from build123d import *

# Parameters (mm, degrees)
SKETCH_1_W      = 33
SKETCH_1_H      = 16
SKETCH_1_R      = 1.7
EXTRUDE_1_DEPTH = 5
EXTRUDE_2_DEPTH = 2.65
SKETCH_3_W      = 0.8
SKETCH_3_H      = 5
EXTRUDE_3_DEPTH = 10
CHAMFER_1_SIZE  = 0.6


with BuildPart() as part:
    # 草图1 → 凸台-拉伸1 (new, symmetric)
    with BuildSketch(Plane(origin=(0, 0, 0), x_dir=(1, 0, 0), z_dir=(0, 1, 0))):
        Rectangle(SKETCH_1_W, SKETCH_1_H)
        with Locations(Location((-11.1, 5, 0), (0, 0, 270))):
            Circle(SKETCH_1_R, mode=Mode.SUBTRACT)
        with Locations(Location((11.1, -5, 0), (0, 0, 270))):
            Circle(SKETCH_1_R, mode=Mode.SUBTRACT)
    extrude(amount=EXTRUDE_1_DEPTH, both=True)

    # 草图2 → 凸台-拉伸2 (add, symmetric)
    with BuildSketch(Plane(origin=(0, 0, 0), x_dir=(1, 0, 0), z_dir=(0, 1, 0))):
        with BuildLine():
            Line((3.236985687, -9.8), (-13.498945121, -9.8))
            Line((-13.498945121, -9.8), (-13.498945121, -10.3))
            Line((-13.498945121, -10.3), (-2.457771256, -10.3))
            Line((-2.457771256, -10.3), (-13.404349416, -11.402516894))
            Line((-13.404349416, -11.402516894), (-13.354243938, -11.9))
            Line((-13.354243938, -11.9), (6.231752422, -9.92733863))
            Line((6.231752422, -9.92733863), (6.231752422, -4.606941304))
            ThreePointArc((6.231752422, -4.606941304), (4.679221154, -3.232884233), (3.236985687, -4.72229453))
            Line((3.236985687, -4.72229453), (3.236985687, -9.8))
        make_face()
    extrude(amount=EXTRUDE_2_DEPTH, both=True)

    # 草图3 → 凸台-拉伸3 (add)
    with BuildSketch(Plane(origin=(16.5, 0, 0), x_dir=(0, 0, -1), z_dir=(1, 0, 0))):
        with Locations((-3.8, 0)):
            Rectangle(SKETCH_3_W, SKETCH_3_H)
        Rectangle(SKETCH_3_W, SKETCH_3_H)
        with Locations((3.8, 0)):
            Rectangle(SKETCH_3_W, SKETCH_3_H)
    extrude(amount=EXTRUDE_3_DEPTH)

    # 倒角1
    chamfer_1_edges = [part.edges().sort_by_distance(p)[0] for p in [
        (26.5, -2.5, 3.8),
        (26.5, 2.5, 3.8),
        (26.5, -2.5, 0),
        (26.5, 2.5, 0),
        (-16.5, 0, -8),
        (26.5, -2.5, -3.8),
        (16.5, 0, -8),
        (26.5, 2.5, -3.8),
        (16.5, 0, 8),
        (-16.5, 0, 8),
    ]]
    chamfer(chamfer_1_edges, length=CHAMFER_1_SIZE)


solid = part.part
Source: CAD feature listing. Evaluate the final solid. Frame: model axes, mm. A direction names the side the tool comes from. Round coordinates to 2 decimals unless told otherwise and drop trailing zeros. Order: outer loops, then holes, each group sorted by start corner. A loop starts at its lowest first (then second) coordinate and runs counter-clockwise, first axis right, second up. Notation, with made-up numbers: (-19.5, 42.5) - (5.5, 42.5) arc R20 ccw to (5.5, 65.5) - close; hole circle Ø7 at (32.25, 40.5). An arc over 180 degrees is marked (long way). Use a Markdown table: item, result. Add a question column.
1. Section query D-D (z = 5). Return the cut outline in (x, y).
2. Section query A-A (x = 24.5). Return the cut outline in (y, z).
3. Section query B-B (x = 11.1). Return the cut outline in (y, z), then the cut area to 3 significant figures.
4. Section query C-C (y = 0.5). Give the number of separate pieces and of enclosed holes in the cut face, then the cut area to 3 significant figures.
5. First-contact query: pin 1 (0.6 mm diameter, centred on y = 1.5, z = 10, fed in from -X); pin 2 (1.5 mm diameter, centred on x = 21, y = 0.5, fed in from +Z); pin 3 (0.9 mm diameter, centred on x = 22, z = 3.5, fed in from +Y). Flat tips, straight axial feed; report the tip coordinate or a pass-through.
6. Set-up query: faces 1 (the flat face through (3.237, 0, 9)), 2 (the flat face through (21, 2.5, 4)), 3 (the flat face through (21, 0, -0.4)), 4 (the flat face through (-3, -2.65, 10)). Return all of +Z, -Z, +X, -X, +Y, -Y with unobstructed straight access to the full face (end or side cutting, diameter ignored); none if empty.
7. Line query: probe 1 along X at (y, z) = (0.25, -5); probe 2 along Z at (x, y) = (-9, -2); probe 3 along X at (y, z) = (-1, 7). Output: solid intervals per line, ascending.
8. Mould query, pull axis Z, two halves, no side actions, for faces 5 (the flat face through (26.5, 0, -4)), 6 (the flat face through (-7.854, 0.037, 10.844)), 7 (the flat face through (21, 0, 4.2)). Classes: +Z half, -Z half, draft (parallel to the pull), parting line (faces both ways), or undercut.
Derived:
| question | item | result |
|---|---|---|
| 1 | outline | (-16.5, -5) - (9.4, -5) - (9.4, 5) - (-16.5, 5) - close; (12.8, -5) - (16.5, -5) - (16.5, 5) - (12.8, 5) - close |
| 2 | outline | (-2.5, -4.2) - (2.5, -4.2) - (2.5, -3.4) - (-2.5, -3.4) - close; (-2.5, -0.4) - (2.5, -0.4) - (2.5, 0.4) - (-2.5, 0.4) - close; (-2.5, 3.4) - (2.5, 3.4) - (2.5, 4.2) - (-2.5, 4.2) - close |
| 3 | outline | (-5, -8) - (5, -8) - (5, 3.3) - (-5, 3.3) - close; (-5, 6.7) - (5, 6.7) - (5, 8) - (-5, 8) - close |
| 3 | area | 126 mm2 |
| 4 | separate pieces | 1 |
| 4 | enclosed holes | 2 |
| 4 | area | 554 mm2 |
| 5 | pin 1 | x = -13.5 |
| 5 | pin 2 | z = 4.2 |
| 5 | pin 3 | y = 2.5 |
| 6 | face 1 | -X, +Y, -Y |
| 6 | face 2 | +Z, -Z, +X, +Y |
| 6 | face 3 | +X, +Y, -Y |
| 6 | face 4 | +Z, +X, -X, -Y |
| 7 | probe 1 | -16.5 to -12.8, -9.4 to 16.5 |
| 7 | probe 2 | -8 to 8, 9.8 to 10.3, 10.96 to 11.46 |
| 7 | probe 3 | -16.5 to 16.5 |
| 8 | face 5 | draft |
| 8 | face 6 | undercut |
| 8 | face 7 | +Z half |
